Autodesk Inventor part; units mm, degrees
ref_plane "YZ Plane" through (0, 0, 0) normal (1, 0, 0) x (0, 1, 0)
ref_plane "XZ Plane" through (0, 0, 0) normal (0, 1, 0) x (-1, 0, 0)
ref_plane "XY Plane" through (0, 0, 0) normal (0, 0, 1) x (1, 0, 0)
sketch "Sketch1" plane through (0, 0, 0) normal (0, 0, 1) x (1, 0, 0)
  circle A0 centre (0, 0) radius 8.5
  circle A1 centre (0, 0) radius 35
  dimension "d0" = 17
  dimension "d1" = 70
extrude "Extrusion1" add sketch "Sketch1" along normal blind 10
sketch "Sketch2" plane through (0, 0, 10) normal (0, 0, 1) x (1, 0, 0)
  circle A0 centre (0, 28) radius 2.2143
  point P0 (0, 0)
  dimension "d4" = 28
hole "Hole1" at (0, 28, 10) direction (0, 0, -1) diameter 5.2 end through all
thread "Thread1"
pattern_circular "Circular Pattern1" count 8 over 360 about axis through (0, 0, 0) along (0, 0, 1) of "Hole1"
properties part number "Nose Hub"
Can you work these out from the model? Positions are in its coordinate system, mm. Round coordinates to 2 decimals unless told otherwise and drop trailing zeros. Write each loop counter-clockwise with the first axis right and the second up, starting at its lowest first coordinate (ties: lowest second). Pieces come first, ordered by that corner, then holes. Notation, with made-up numbers: M 73.25,89.25 L 125.25,89.25 A24 ccw 125.25,110.25 Z; hole C 24.25,11.25 d1. An arc over 180 degrees is marked long. Use a Markdown table: item, result.
Item 1: For pin 1 Ø3 at (x, y) = (19.8, 19.8) entering from +Z; pin 2 Ø1 at (x, z) = (-8, 3) entering from +Y; pin 3 Ø3 at (x, z) = (-3.5, 8.5) entering from -Y, each with a flat end and sliding along its axis, tell me the tip position at first contact or that it passes through.
Found:
| item | result |
|---|---|
| pin 1 | passes through |
| pin 2 | stops at y = 34.19 |
| pin 3 | stops at y = -34.94 |
Item 2: I want a section at A-A (x = 0). List the corners of the cut face in (y, z) for me, and give its area (3 significant figures).
Found:
| item | result |
|---|---|
| outline | M -35,0 L -30.6,0 L -30.6,10 L -35,10 Z; M -25.4,0 L -8.5,0 L -8.5,10 L -25.4,10 Z; M 8.5,0 L 25.4,0 L 25.4,10 L 8.5,10 Z; M 30.6,0 L 35,0 L 35,10 L 30.6,10 Z |
| area | 426 mm2 |
Item 3: We'd pull the mould along Y, two halves only. Please class faces 1 (the face through (-28, 21, 5)), 2 (the face through (7, -7, 10)), 3 (the face through (0.1, -30.6, 4.9)): released by +Y, released by -Y, zero draft, split by the parting line, or undercut.
Found:
| item | result |
|---|---|
| face 1 | split by the parting line |
| face 2 | zero draft |
| face 3 | undercut |
Item 4: If I drill on line 1 along Y through (x, z) = (-19, 8); line 2 along X through (y, z) = (1, 1.25); line 3 along X through (y, z) = (-22, 8.75), over which ranges is the centre line in solid material (lowest first)? Write a range as [from, to].
Found:
| item | result |
|---|---|
| line 1 | y = [-29.39, -22.27], [-17.32, 17.32], [22.27, 29.39] |
| line 2 | x = [-34.99, -30.4], [-25.6, -8.44], [8.44, 25.6], [30.4, 34.99] |
| line 3 | x = [-27.22, -21.18], [-18.41, 18.41], [21.18, 27.22] |
Item 5: I want a section at B-B (y = 28). List the corners of the cut face in (x, z) for me, and give its area (3 significant figures).
Found:
| item | result |
|---|---|
| outline | M -21,0 L -2.6,0 L -2.6,10 L -21,10 Z; M 2.6,0 L 21,0 L 21,10 L 2.6,10 Z |
| area | 368 mm2 |
